from build123d import *

# Parameters (mm, degrees)
SKETCH2_W           = 190.5
SKETCH2_H           = 203.2
BOSS_EXTRUDE1_DEPTH = 6
SKETCH5_R           = 2.5
CUT_EXTRUDE6_DEPTH  = 7
CUT_EXTRUDE7_DEPTH  = 10


with BuildPart() as part:
    # Sketch2 → Boss-Extrude1 (new body)
    with BuildSketch(Plane(origin=(0, 0, 0), x_dir=(1, 0, 0), z_dir=(0, 1, 0))):
        Rectangle(SKETCH2_W, SKETCH2_H)
    extrude(amount=BOSS_EXTRUDE1_DEPTH)

    # Sketch5 → Cut-Extrude6 (cut, through all)
    with BuildSketch(Plane(origin=(0, 6, 0), x_dir=(1, 0, 0), z_dir=(0, 1, 0))):
        with Locations((-78.187036158, 94.165073798)):
            Circle(SKETCH5_R)
        with Locations((0, 94.165073798)):
            Circle(SKETCH5_R)
        with Locations((78.187036158, 0)):
            Circle(SKETCH5_R)
        with Locations((-78.187036158, 0)):
            Circle(SKETCH5_R)
        with Locations((78.187036158, 94.165073798)):
            Circle(SKETCH5_R)
        with Locations((-78.187036158, -94.165073798)):
            Circle(SKETCH5_R)
        with Locations((78.187036158, -94.165073798)):
            Circle(SKETCH5_R)
    extrude(amount=-CUT_EXTRUDE6_DEPTH, mode=Mode.SUBTRACT)

    # Sketch6 → Cut-Extrude7 (cut)
    with BuildSketch(Plane(origin=(0, 6, 0), x_dir=(1, 0, 0), z_dir=(0, 1, 0))):
        with BuildLine():
            ThreePointArc((-13.95, 74.35), (-17.364213562, 75.764213562), (-15.95, 72.35))
            Line((-15.95, 72.35), (-15.95, 74.35))
            Line((-15.95, 74.35), (-13.95, 74.35))
        make_face()
        with BuildLine():
            Line((-15.95, 74.35), (-15.95, 72.35))
            ThreePointArc((-15.95, 72.35), (-14.535786438, 72.935786438), (-13.95, 74.35))
            Line((-13.95, 74.35), (-15.95, 74.35))
        make_face()
        with BuildLine():
            ThreePointArc((13.95, 74.35), (14.535786438, 72.935786438), (15.95, 72.35))
            Line((15.95, 72.35), (15.95, 74.35))
            Line((15.95, 74.35), (13.95, 74.35))
        make_face()
        with BuildLine():
            Line((15.95, 74.35), (15.95, 72.35))
            ThreePointArc((15.95, 72.35), (17.364213562, 72.935786438), (17.95, 74.35))
            ThreePointArc((17.95, 74.35), (15.95, 76.35), (13.95, 74.35))
            Line((13.95, 74.35), (15.95, 74.35))
        make_face()
        with BuildLine():
            Line((-15.95, 44.45), (-15.95, 42.45))
            Line((-15.95, 42.45), (-13.95, 42.45))
            ThreePointArc((-13.95, 42.45), (-14.535786438, 43.864213562), (-15.95, 44.45))
        make_face()
        with BuildLine():
            ThreePointArc((-15.95, 44.45), (-17.95, 42.45), (-15.95, 40.45))
            Line((-15.95, 40.45), (-15.95, 42.45))
            Line((-15.95, 42.45), (-15.95, 44.45))
        make_face()
        with BuildLine():
            ThreePointArc((15.95, 44.45), (14.535786438, 43.864213562), (13.95, 42.45))
            Line((13.95, 42.45), (15.95, 42.45))
            Line((15.95, 42.45), (15.95, 44.45))
        make_face()
        with BuildLine():
            Line((15.95, 42.45), (17.95, 42.45))
            ThreePointArc((17.95, 42.45), (17.364213562, 43.864213562), (15.95, 44.45))
            Line((15.95, 44.45), (15.95, 42.45))
        make_face()
        with BuildLine():
            ThreePointArc((13.95, 42.45), (15.95, 40.45), (17.95, 42.45))
            Line((17.95, 42.45), (15.95, 42.45))
            Line((15.95, 42.45), (13.95, 42.45))
        make_face()
        with BuildLine():
            Line((-15.95, 42.45), (-15.95, 40.45))
            ThreePointArc((-15.95, 40.45), (-14.535786438, 41.035786438), (-13.95, 42.45))
            Line((-13.95, 42.45), (-15.95, 42.45))
        make_face()
        Polygon((-55.95, 11), (-55.95, 0), (-24.05, 0), (-24.05, 11), (-40, 11), align=None)
        Polygon((40, 0), (55.95, 0), (55.95, 11), (40, 11), (24.05, 11), (24.05, 0), align=None)
    extrude(amount=-CUT_EXTRUDE7_DEPTH, mode=Mode.SUBTRACT)


solid = part.part
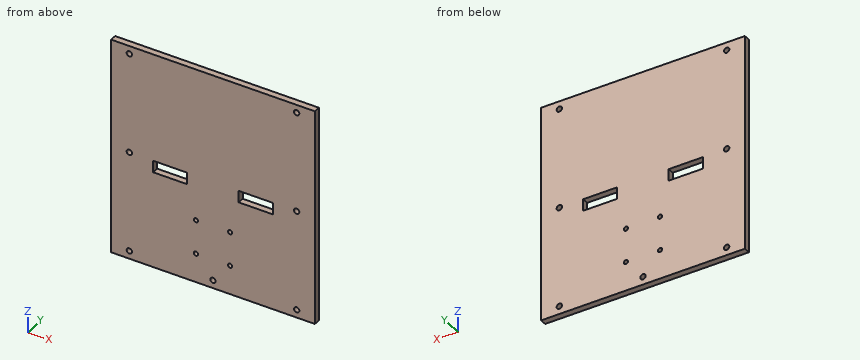
Build history of the part. All positions in model axes, mm. Coordinates: 2 decimals unless noted, no trailing zeros. Order: outer loops, then holes, each group sorted by start corner. A loop starts at its lowest first (then second) coordinate and runs counter-clockwise, first axis right, second up. Notation, with made-up numbers: M 45,68 L 89,68 A27 ccw 89,92 Z; hole C -22.5,-9 d9. An arc over 180 degrees is marked long. One line per question, with ' | ' between items. Start each with the question number.
Q1. Probe L1, parallel to X at y = 2.7, z = -74.35; L2, parallel to X at y = 3.6, z = -10.5; L3, parallel to Z at x = 32, y = 5.55. List the from-to ranges inside material, lowest first. Write a range as from..to.
Q2. Saw through at B-B (y = 1.55). Count the separate pieces of the cut face and the enclosed holes in it, then the cut area to 3 significant figures.
Q3. Saw through at A-A (x = 0). List the corners of the cut face in (y, z), then the cut area to 3 significant figures.
Check values:
1) L1: x = -95.25..-17.95, -13.95..13.95, 17.95..95.25 | L2: x = -95.25..-55.95, -24.05..24.05, 55.95..95.25 | L3: z = -101.6..-11, 0..101.6
2) separate pieces: 1 | enclosed holes: 13 | area: 37,800 mm2
3) outline: M 0,-101.6 L 6,-101.6 L 6,-96.67 L 0,-96.67 Z; M 0,-91.67 L 6,-91.67 L 6,101.6 L 0,101.6 Z | area: 1,190 mm2
